The model under review builds one solid part; all positions refer to its coordinate system, in mm. A direction names the side the tool comes from. Give positions to 0.01 mm unless a question says otherwise; leave off trailing zeros. Write each loop counter-clockwise with the first axis right and the second up, starting at its lowest first coordinate (ties: lowest second). Pieces come first, ordered by that corner, then holes. Notation, with made-up numbers: M 84,-23 L 98,-23 A33 ccw 98,9 Z; hole C 27,-36.5 d7. An arc over 180 degrees is marked long. Write item = value, one per line. Start each with the question number.
```python
from build123d import *

# Parameters (mm, degrees)
F1_DEPTH  = 20
F2_R      = 12.5
F3_DEPTH  = 210.001
F4_R      = 19
F4_R_2    = 14
F5_DEPTH  = 2.7
F6_R      = 19
F6_R_2    = 14
F7_DEPTH  = 2.7
F9_DEPTH  = 2.7
F11_DEPTH = 2.7
F12_R     = 2.5
F13_DEPTH = 10
F14_R     = 2.5
F15_DEPTH = 10
F16_R     = 6.5
F17_DEPTH = 20
F18_R     = 4.25
F19_DEPTH = 40.0010001
F20_R     = 3
F21_DEPTH = 10
F24_W     = 1.5
F24_H     = 28.0618912584
F26_W     = 24.1605055332
F26_H     = 1.5
F28_R     = 5
F29_DEPTH = 40.0010001
F30_R     = 4
F31_DEPTH = 16


# Not quite as in the source:
# - a pattern or mirror of a feature is missing from the dataset's text; its kind, count and spacing are read off the source's solid


with BuildPart() as f1:
    # F0 (on Front) → F1 (new body, symmetric)
    with BuildSketch(Plane.XZ):
        Polygon((80, 150), (-80, 150), (-105, 125), (-105, -125), (-80, -150), (80, -150), (105, -125), (105, 125), align=None)
        with BuildLine():
            ThreePointArc((-54.6611964743, 0), (0, 124.08), (54.6611964743, 0))
            ThreePointArc((54.6611964743, 0), (0, -124.08), (-54.6611964743, 0))
        make_face(mode=Mode.SUBTRACT)
    extrude(amount=F1_DEPTH, both=True)

    # F2 (on face) → F3 (cut, through all)
    with BuildSketch(Plane.YZ.offset(105)):
        Circle(F2_R)
    extrude(amount=-F3_DEPTH, mode=Mode.SUBTRACT)

    # F4 (on face) → F5 (cut)
    with BuildSketch(Plane.YZ.offset(105)):
        Circle(F4_R)
        Circle(F4_R_2, mode=Mode.SUBTRACT)
    extrude(amount=-F5_DEPTH, mode=Mode.SUBTRACT)

    # F6 (on face) → F7 (cut)
    with BuildSketch(Plane(origin=(-105, 0, 0), x_dir=(0, -1, 0), z_dir=(-1, 0, 0))):
        Circle(F6_R)
        Circle(F6_R_2, mode=Mode.SUBTRACT)
    extrude(amount=-F7_DEPTH, mode=Mode.SUBTRACT)

    # F8 (on face) → F9 (cut)
    with BuildSketch(Plane(origin=(0, 20, 0), x_dir=(-1, 0, 0), z_dir=(0, 1, 0))):
        with BuildLine():
            ThreePointArc((-69.9714227381, 0), (0, -136), (69.9714227381, 0))
            ThreePointArc((69.9714227381, 0), (0, 136), (-69.9714227381, 0))
        make_face()
        with BuildLine():
            ThreePointArc((0, 131), (72.8388632531, 85.4330354331), (63.7259758654, 0))
            ThreePointArc((63.7259758654, 0), (72.8388632531, -85.4330354331), (0, -131))
            ThreePointArc((0, -131), (-72.8388632531, -85.4330354331), (-63.7259758654, 0))
            ThreePointArc((-63.7259758654, 0), (-72.8388632531, 85.4330354331), (0, 131))
        make_face(mode=Mode.SUBTRACT)
    extrude(amount=-F9_DEPTH, mode=Mode.SUBTRACT)

    # F10 (on face) → F11 (cut)
    with BuildSketch(Plane.XZ.offset(20)):
        with BuildLine():
            ThreePointArc((69.9714227381, 0), (0, 136), (-69.9714227381, 0))
            ThreePointArc((-69.9714227381, 0), (0, -136), (69.9714227381, 0))
        make_face()
        with BuildLine():
            ThreePointArc((0, 131), (72.8388632531, 85.4330354331), (63.7259758654, 0))
            ThreePointArc((63.7259758654, 0), (72.8388632531, -85.4330354331), (0, -131))
            ThreePointArc((0, -131), (-72.8388632531, -85.4330354331), (-63.7259758654, 0))
            ThreePointArc((-63.7259758654, 0), (-72.8388632531, 85.4330354331), (0, 131))
        make_face(mode=Mode.SUBTRACT)
    extrude(amount=-F11_DEPTH, mode=Mode.SUBTRACT)

    # F12 (on face) → F13 (cut)
    with BuildSketch(Plane.YZ.offset(105)):
        with Locations((-15, 20)):
            Circle(F12_R)
        with Locations((15, 20)):
            Circle(F12_R)
        with Locations((15, -20)):
            Circle(F12_R)
        with Locations((-15, -20)):
            Circle(F12_R)
    extrude(amount=-F13_DEPTH, mode=Mode.SUBTRACT)

    # F14 (on face) → F15 (cut)
    with BuildSketch(Plane(origin=(-105, 0, 0), x_dir=(0, -1, 0), z_dir=(-1, 0, 0))):
        with Locations((-15, 20)):
            Circle(F14_R)
        with Locations((15, 20)):
            Circle(F14_R)
        with Locations((15, -20)):
            Circle(F14_R)
        with Locations((-15, -20)):
            Circle(F14_R)
    extrude(amount=-F15_DEPTH, mode=Mode.SUBTRACT)

    # F16 (on face) → F17 (cut)
    with BuildSketch(Plane.XZ.offset(20)):
        with Locations((-50, 140)):
            Circle(F16_R)
        with Locations((50, 140)):
            Circle(F16_R)
        with Locations((-50, -140)):
            Circle(F16_R)
        with Locations((50, -140)):
            Circle(F16_R)
        with Locations((95, 70)):
            Circle(F16_R)
        with Locations((95, -70)):
            Circle(F16_R)
        with Locations((-95, 70)):
            Circle(F16_R)
        with Locations((-95, -70)):
            Circle(F16_R)
    extrude(amount=-F17_DEPTH, mode=Mode.SUBTRACT)

    # F18 (on face) → F19 (cut, through all)
    with BuildSketch(Plane.XZ.offset(20)):
        with Locations((-50, 140)):
            Circle(F18_R)
        with Locations((50, 140)):
            Circle(F18_R)
        with Locations((95, 70)):
            Circle(F18_R)
        with Locations((95, -70)):
            Circle(F18_R)
        with Locations((50, -140)):
            Circle(F18_R)
        with Locations((-50, -140)):
            Circle(F18_R)
        with Locations((-95, -70)):
            Circle(F18_R)
        with Locations((-95, 70)):
            Circle(F18_R)
    extrude(amount=-F19_DEPTH, mode=Mode.SUBTRACT)

    # F20 (on face) → F21 (cut)
    with BuildSketch(Plane.XZ.offset(20)):
        with Locations((0, 145)):
            Circle(F20_R)
        with Locations((-95, 50)):
            Circle(F20_R)
        with Locations((-95, -50)):
            Circle(F20_R)
        with Locations((95, -50)):
            Circle(F20_R)
        with Locations((95, 50)):
            Circle(F20_R)
        with Locations((0, -145)):
            Circle(F20_R)
    extrude(amount=-F21_DEPTH, mode=Mode.SUBTRACT)

    # F22 (on Front) → F23 (revolve, cut)
    with BuildSketch(Plane.XZ):
        Polygon((-89.6732207666, 140.3267792334), (-92.5016478914, 137.4983521086), (-85.4305800795, 130.4272842968), (-84.3699199077, 131.4879444685), (-82.6021529548, 133.2557114215), align=None)
        Polygon((-84.3699199077, 131.4879444685), (-85.4305800795, 130.4272842968), (-49.1876475233, 94.1843517405), (-48.1269873515, 95.2450119123), align=None)
    f23 = revolve(axis=Axis((-46.2508239457, 0, 91.2475281629), (0.7071067812, 0, -0.7071067812)), mode=Mode.SUBTRACT)

    # F23_copies: F23 across plane
    add(f23.mirror(Plane(origin=(6e-06, 0, 0), x_dir=(0, 0, 1), z_dir=(1, 0, 0))), mode=Mode.SUBTRACT)

    # F24 (on Front) → F25 (revolve, cut)
    with BuildSketch(Plane.XZ):
        with Locations((0.75, 125.9690543708)):
            Rectangle(F24_W, F24_H)
        Polygon((0, 162.6632596409), (0, 140), (1.5, 140), (4, 140), (4, 162.6632596409), align=None)
    revolve(axis=Axis((0, 0, 81.3316298204), (0, 0, 1)), mode=Mode.SUBTRACT)

    # F26 (on Front) → F27 (revolve, cut)
    with BuildSketch(Plane.XZ):
        with Locations((82.9197472334, 49.25)):
            Rectangle(F26_W, F26_H)
        Polygon((111.5470026106, 50), (95, 50), (95, 48.5), (95, 46), (111.5470026106, 46), align=None)
    f27 = revolve(axis=Axis((9.1493800282, 0, 50), (1, 0, 0)), mode=Mode.SUBTRACT)

    # F27_copies: F27 across plane
    add(f27.mirror(Plane(origin=(1e-06, 0, 0), x_dir=(0, 0, -1), z_dir=(-1, 0, 0))), mode=Mode.SUBTRACT)

    # F28 (on face) → F29 (cut, through all)
    with BuildSketch(Plane.XZ.offset(20)):
        with Locations((70, 140)):
            Circle(F28_R)
        with Locations((-70, -140)):
            Circle(F28_R)
    extrude(amount=-F29_DEPTH, mode=Mode.SUBTRACT)

    # F30 (on face) → F31 (cut)
    with BuildSketch(Plane.XZ.offset(20)):
        with Locations((-90, 120)):
            Circle(F30_R)
        with Locations((90, 120)):
            Circle(F30_R)
        with Locations((90, -120)):
            Circle(F30_R)
        with Locations((-90, -120)):
            Circle(F30_R)
    extrude(amount=-F31_DEPTH, mode=Mode.SUBTRACT)


solid = f1.part
```
Item 1: Clearance check with flat-ended pins moving along their axes: P1, Ø5, axis at x = 90, z = 120, coming from the -Y side; P2, Ø1.5, axis at y = 15.5, z = 19, coming from the +X side; P3, Ø5, axis at y = 0, z = 50, coming from the -X side. State where each tip first meets the part, or that it passes through.
Item 2: For faces 1 (the flat face through (96.4, 0, 65.8)), 2 (the cylindrical face through (-2.64, 18.67, 135.96)), 3 (the flat face through (102.3, -9, -11)), list the 3-axis set-ups (+Z, -Z, +X, -X, +Y, -Y) from which the entire face can be reached by the end or side of a thin tool; tool diameter is ignored.
Item 3: We need section A-A, the plane x = -21. Write out the cut boundary in (y, z), and give its area (3 significant figures).
Item 4: We need section B-B, the plane x = 17.5. Write out the cut boundary in (y, z).
Item 5: The part is to be moulded in two halves that separate along Y. For faces 4 (the cylindrical face through (-98.37, 9.86, -72.59)), 5 (the cylindrical face through (-103.669, -12.932, -5.362)), 6 (the flat face through (95, -10, 50)), say which applies: released by +Y, released by -Y, zero draft, split by the parting line, or undercut.
Item 6: To check wall thickness, follow probe 1 along Z at (x, y) = (95, 18); probe 2 along X at (y, z) = (-17.5, -96.5); probe 3 along Z at (x, y) = (50, 15.25). State the ranges of each line that lie inside material, in increasing order. Write a range as [from, to].
Item 7: We need section C-C, the plane z = 70. Give the number of separate pieces and of enclosed holes in the cut face, and give its area (3 significant figures).
Worked out:
q1.P1 = -4
q1.P2 = 95
q1.P3 = -95
q2.face_1 = -Y
q2.face_2 = +Y
q2.face_3 = +X
q3.outline = M -20,-150 L 20,-150 L 20,-133.4 L 17.3,-133.4 L 17.3,-128.23 L 20,-128.23 L 20,-121.04 L -20,-121.04 L -20,-128.23 L -17.3,-128.23 L -17.3,-133.4 L -20,-133.4 Z; M -20,121.04 L 20,121.04 L 20,128.23 L 17.3,128.23 L 17.3,133.4 L 20,133.4 L 20,150 L -20,150 L -20,133.4 L -17.3,133.4 L -17.3,128.23 L -20,128.23 Z
q3.area = 2,260 mm²
q4.outline = M -20,-150 L 20,-150 L 20,-134.2 L 17.3,-134.2 L 17.3,-129.09 L 20,-129.09 L 20,-121.98 L -20,-121.98 L -20,-129.09 L -17.3,-129.09 L -17.3,-134.2 L -20,-134.2 Z; M -20,121.98 L 20,121.98 L 20,129.09 L 17.3,129.09 L 17.3,134.2 L 20,134.2 L 20,150 L -20,150 L -20,134.2 L -17.3,134.2 L -17.3,129.09 L -20,129.09 Z
q5.face_4 = zero draft
q5.face_5 = undercut
q5.face_6 = released by -Y
q6.probe_1 = [-135, -74.25], [-65.75, 65.75], [74.25, 135]
q6.probe_2 = [-105, -72.34], [-66.32, -57.67], [57.67, 66.32], [72.34, 105]
q6.probe_3 = [-150, -144.25], [-135.75, -104.66], [104.66, 135.75], [144.25, 150]
q7.separate_pieces = 4
q7.enclosed_holes = 0
q7.area = 1,780 mm²
